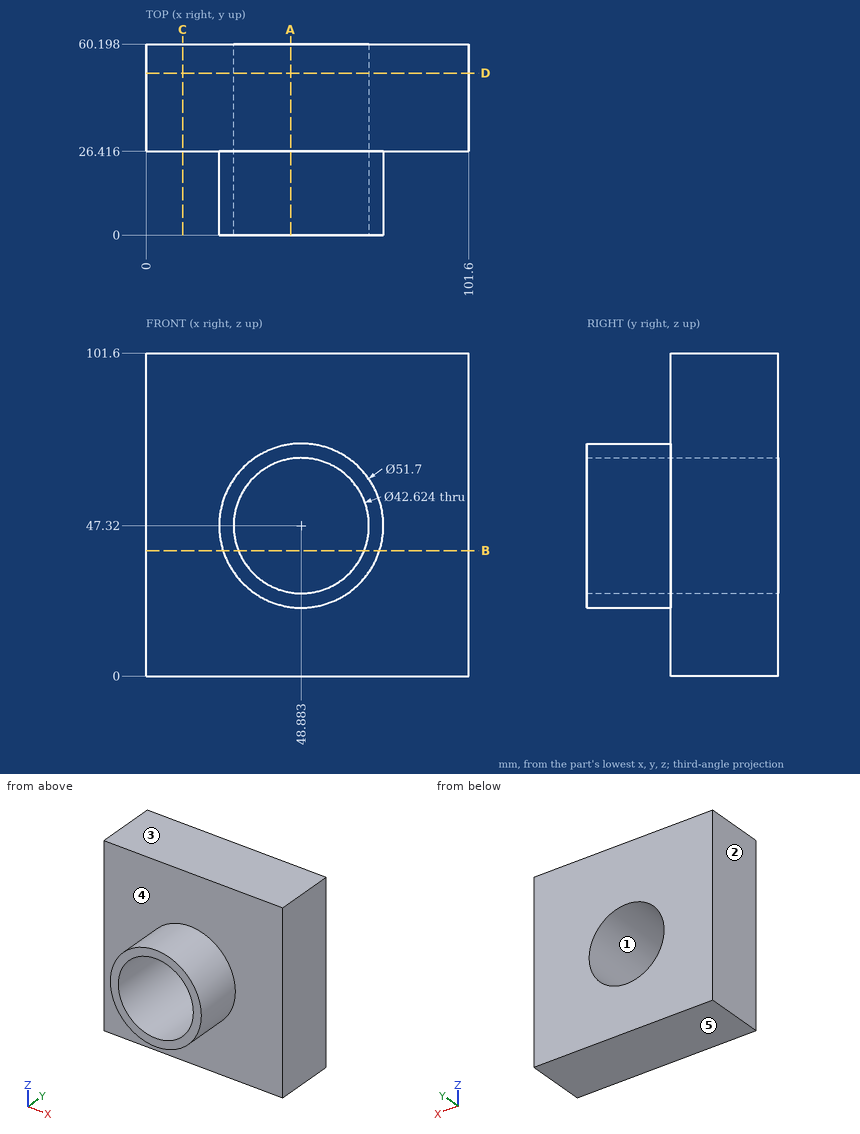
Can you work these out from the drawing? Everything is in mm from the part's minimum corner. A direction names the side the tool comes from. Round coordinates to 2 decimals unless told otherwise and drop trailing zeros. Write each loop counter-clockwise with the first axis right and the second up, starting at its lowest first coordinate (ties: lowest second). Pieces come first, ordered by that corner, then holes. Notation, with made-up numbers: (-22.5, 68.5) - (11.5, 68.5) arc R20 cw to (11.5, 84.5) - close; hole circle Ø5 at (49.25, 1). An arc over 180 degrees is marked (long way). Use a Markdown table: item, result.
Q1. Please list where these lines run through material, in increasing order: L1, parallel to Z at x = 48, y = 57; L2, parallel to Y at x = 63, z = 70; L3, parallel to X at y = 47, z = 31.5 (1 decimal).
Output values:
| item | result |
|---|---|
| L1 | 0 to 26.03, 68.61 to 101.6 |
| L2 | 26.42 to 60.2 |
| L3 | 0 to 34.6, 63.2 to 101.6 |
Q2. Thinking about a two-plate mould opening in Z: for the marked faces 1, 2 and 3, which applies, released by +Z, released by -Z, zero draft, split by the parting line, or undercut?
Output values:
| item | result |
|---|---|
| face 1 | undercut |
| face 2 | zero draft |
| face 3 | released by +Z |
Q3. For the marked faces 4 and 5, which set-ups out of +Z, -Z, +X, -X, +Y, -Y let a thin tool reach every point of the face, with its end or its side?
Output values:
| item | result |
|---|---|
| face 4 | -Y |
| face 5 | -Z, +X, -X, +Y, -Y |
Q4. For pin 1 (10 mm diameter, centred on y = 20, z = 73, fed in from +X) (1 decimal); pin 2 (1 mm diameter, centred on y = 25, z = 35.5, fed in from +X); pin 3 (1.5 mm diameter, centred on x = 37.5, y = 14.5, fed in from -Z), each with a flat end and sliding along its axis, tell me the tip position at first contact or that it passes through.
Output values:
| item | result |
|---|---|
| pin 1 | x = 64.4 |
| pin 2 | x = 72.12 |
| pin 3 | z = 23.76 |
Q5. I want a section at C-C (x = 11.5). List the corners of the cut face in (y, z) for me.
Output values:
| item | result |
|---|---|
| outline | (26.42, 0) - (60.2, 0) - (60.2, 101.6) - (26.42, 101.6) - close |
Q6. I want a section at B-B (z = 39.5). List the corners of the cut face in (x, y) for me (1 decimal), plus the area to 3 significant figures.
Output values:
| item | result |
|---|---|
| outline | (0, 26.4) - (24.2, 26.4) - (24.2, 0) - (29.1, 0) - (29.1, 60.2) - (0, 60.2) - close; (68.7, 0) - (73.5, 0) - (73.5, 26.4) - (101.6, 26.4) - (101.6, 60.2) - (68.7, 60.2) - close |
| area | 2,350 mm2 |
Q7. I want a section at D-D (y = 51). List the corners of the cut face in (x, z) for me (1 decimal), plus the area to 3 significant figures.
Output values:
| item | result |
|---|---|
| outline | (0, 0) - (101.6, 0) - (101.6, 101.6) - (0, 101.6) - close; hole circle Ø42.6 at (48.9, 47.3) |
| area | 8,900 mm2 |
Q8. I want a section at A-A (x = 45.5). List the corners of the cut face in (y, z) for me, plus the area to 3 significant figures.
Output values:
| item | result |
|---|---|
| outline | (0, 21.69) - (26.42, 21.69) - (26.42, 0) - (60.2, 0) - (60.2, 26.28) - (0, 26.28) - close; (0, 68.36) - (60.2, 68.36) - (60.2, 101.6) - (26.42, 101.6) - (26.42, 72.95) - (0, 72.95) - close |
| area | 2,250 mm2 |
